```python
from build123d import *

# Parameters (mm, degrees)
SKETCH_R        = 25
PAD_DEPTH       = 15
SKETCH001_R     = 6.2
POCKET_DEPTH    = 15
SKETCH002_R     = 13
POCKET001_DEPTH = 8


with BuildPart() as part:
    # Sketch → Pad (new body)
    with BuildSketch(Plane.XY):
        Circle(SKETCH_R)
    extrude(amount=PAD_DEPTH)

    # Sketch001 (on Face3 of Pad) → Pocket (cut)
    with BuildSketch(Plane.XY.offset(15)):
        Circle(SKETCH001_R)
    extrude(amount=-POCKET_DEPTH, mode=Mode.SUBTRACT)

    # Sketch002 (on Face3 of Pocket) → Pocket001 (cut)
    with BuildSketch(Plane.XY.offset(15)):
        Circle(SKETCH002_R)
    extrude(amount=-POCKET001_DEPTH, mode=Mode.SUBTRACT)


solid = part.part
```
Work out the finished part from the listing and answer in its coordinate system (mm). A direction names the side the tool comes from. Coordinates: 2 decimals unless noted, no trailing zeros. Write each loop counter-clockwise with the first axis right and the second up, starting at its lowest first coordinate (ties: lowest second). Pieces come first, ordered by that corner, then holes.
Q1. Each of these flat-tipped pins is pushed along its axis until it touches: pin 1 Ø14.5 at (x, y) = (0, 0) entering from +Z; pin 2 Ø1.5 at (y, z) = (9, 9.5) entering from -X; pin 3 Ø1.5 at (x, z) = (-8, 12.5) entering from +Y. Where does it stop, or does it pass through?
Q2. A cutting plane is placed at D-D, the plane z = 3.5. Give the vertices of the cut face in (x, y), then the cut area to 3 significant figures.
Q3. Which of the six approach directions +Z, -Z, +X, -X, +Y, -Y give full straight-line access (tool end or side, diameter ignored) to faces 4 (the face through (6, -3, 7)), 5 (the face through (2.86, -5.5, 3.55))?
Q4. Find the intervals of material crossed by line 1 (Y direction, x = 0, z = 3); line 2 (Y direction, x = 0, z = 12.5); line 3 (Z direction, x = 5, y = -4), in increasing order.
Q5. A cutting plane is placed at C-C, the plane x = 15. Give the vertices of the cut face in (y, z), then the cut area to 3 significant figures.
Q6. Determine the mould class of faces 1 (the face through (5, -5, 0)), 2 (the face through (23.846, 7.509, 7.395)), 3 (the face through (-10.316, -7.91, 11.056)) for opening direction X: released by +X, released by -X, zero draft, split by the parting line, or undercut.
Q7. A cutting plane is placed at A-A, the plane x = 0. Give the vertices of the cut face in (y, z).
Findings below:
1. pin 1: stops at z = 7
1. pin 2: stops at x = -23.6
1. pin 3: stops at y = 23.93
2. outline: circle Ø50 at (0, 0); hole circle Ø12.4 at (0, 0)
2. area: 1,840 mm2
3. face 4: +Z
3. face 5: +Z, -Z
4. line 1: y = -25 to -6.2, 6.2 to 25
4. line 2: y = -25 to -13, 13 to 25
4. line 3: z = 0 to 7
5. outline: (-20, 0) - (20, 0) - (20, 15) - (-20, 15) - close
5. area: 600 mm2
6. face 1: zero draft
6. face 2: split by the parting line
6. face 3: undercut
7. outline: (-25, 0) - (-6.2, 0) - (-6.2, 7) - (-13, 7) - (-13, 15) - (-25, 15) - close; (6.2, 0) - (25, 0) - (25, 15) - (13, 15) - (13, 7) - (6.2, 7) - close
